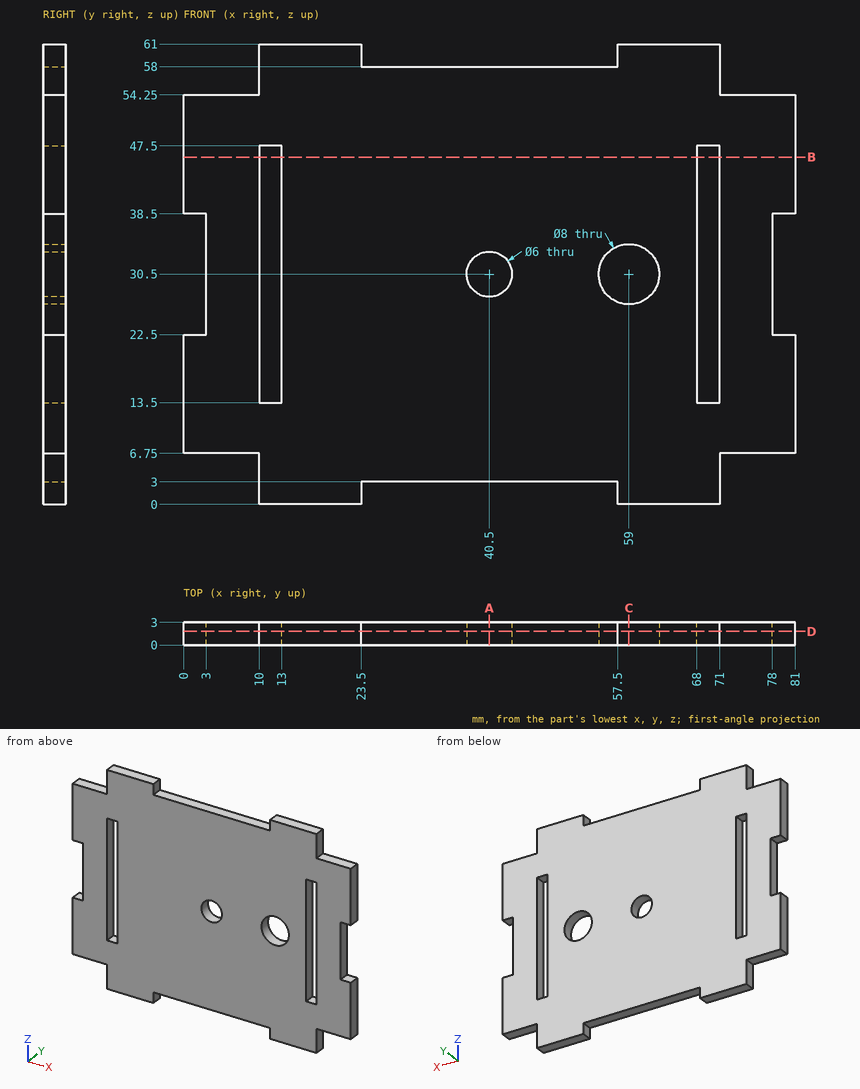
Geometry check sheet. Reference: drawing and pictorial views, mm from the part's lowest x, y, z. Give positions to 0.01 mm unless a question says otherwise; leave off trailing zeros. Loops run counter-clockwise (first coordinate to the right, second up) from the corner with the lowest first, then second, coordinate; pieces in that order, holes last. Notation, with made-up numbers: M -20.5,44 L -5.5,44 A18 ccw -5.5,70 Z; hole C 83.25,52 d3. An arc over 180 degrees is marked long. Use a Markdown table: item, result. Add a question column.
Q1. Sectioned sample at A-A, the plane x = 40.5. Record the cut outline in (y, z), then the cut area to 3 significant figures.
Q2. Scan lines: line 1 along X through (y, z) = (0.8, 23.5); line 2 along X through (y, z) = (2.7, 40.5); line 3 along X through (y, z) = (2.35, 30.5). Record each from-to range of solid material in increasing order. Write a range as [from, to].
Q3. Sectioned sample at C-C, the plane x = 59. Record the cut outline in (y, z), then the cut area to 3 significant figures.
Q4. Sectioned sample at B-B, the plane z = 46. Record the cut outline in (x, y).
Q5. Go/stop test with flat-tipped pins: pin 1 (0.9 mm diameter, centred on y = 1.5, z = 59.5, fed in from +X); pin 2 (1.5 mm diameter, centred on x = 79, y = 1, fed in from +Z). Record where each tip stops, or that it passes through.
Q6. Sectioned sample at D-D, the plane y = 1.8. Give the number of separate pieces and of enclosed holes in the cut face, then the cut area to 3 significant figures.
Verdict:
| question | item | result |
|---|---|---|
| 1 | outline | M 0,3 L 3,3 L 3,27.5 L 0,27.5 Z; M 0,33.5 L 3,33.5 L 3,58 L 0,58 Z |
| 1 | area | 147 mm^2 |
| 2 | line 1 | [3, 10], [13, 68], [71, 78] |
| 2 | line 2 | [0, 10], [13, 68], [71, 81] |
| 2 | line 3 | [3, 10], [13, 37.5], [43.5, 55], [63, 68], [71, 78] |
| 3 | outline | M 0,0 L 3,0 L 3,26.5 L 0,26.5 Z; M 0,34.5 L 3,34.5 L 3,61 L 0,61 Z |
| 3 | area | 159 mm^2 |
| 4 | outline | M 0,0 L 10,0 L 10,3 L 0,3 Z; M 13,0 L 68,0 L 68,3 L 13,3 Z; M 71,0 L 81,0 L 81,3 L 71,3 Z |
| 5 | pin 1 | x = 71 |
| 5 | pin 2 | z = 54.25 |
| 6 | separate pieces | 1 |
| 6 | enclosed holes | 4 |
| 6 | area | 4,090 mm^2 |
